Design review of the part built by this model. Coordinates are the model's own, in mm. A direction names the side the tool comes from. Coordinates: 2 decimals unless noted, no trailing zeros. Loops run counter-clockwise (first coordinate to the right, second up) from the corner with the lowest first, then second, coordinate; pieces in that order, holes last. Notation, with made-up numbers: (71, -16.5) - (104, -16.5) arc R16 ccw to (104, -11.5) - close; hole circle Ø3 at (66.5, 40). An arc over 180 degrees is marked (long way). Answer in a Markdown table with one row per item. Add a question column.
(1) For faces 5 (the face through (-9.75, 4, 0)), 6 (the face through (0, 9, 8)), 7 (the face through (-7.5, 11, 2.8)), list the 3-axis set-ups (+Z, -Z, +X, -X, +Y, -Y) from which the entire face can be reached by the end or side of a thin tool; tool diameter is ignored.
(2) We need section B-B, the plane y = 15.25. Write out the cut boundary in (x, z).
(3) We need section A-A, the plane y = 10.5. Write out the cut boundary in (x, z), plus the area to 3 significant figures.
(4) The part is to be moulded in two halves that separate along Y. For faces 1 (the face through (0, 5, 9.75)), 2 (the face through (0, 10.8, 8.2)), 3 (the face through (0, 10, 6.55)), 4 (the face through (0, 0, 0)), say which applies: released by +Y, released by -Y, zero draft, split by the parting line, or undercut.
(5) Clearance check with flat-ended pins moving along their axes: pin 1 (1.4 mm diameter, centred on x = 0, y = 10, fed in from +Z); pin 2 (1 mm diameter, centred on x = -7, y = 20, fed in from -Z); pin 3 (4 mm diameter, centred on y = 15.5, z = -1.5, fed in from -X). State where each tip first meets the part, or that it passes through.
(6) To check wall thickness, follow L1, parallel to Y at x = 0, z = 8.7; L2, parallel to Y at x = 0, z = 7.4; L3, parallel to Y at x = -5.5, z = 7.5. State the ranges of each line that lie inside material, in increasing order. Write a range as [from, to].
from build123d import *

# Parameters (mm, degrees)
SKETCH1_W           = 19.5
SKETCH1_H           = 19.5
BOSS_EXTRUDE1_DEPTH = 11
SKETCH2_R           = 7.75
BOSS_EXTRUDE2_DEPTH = 9
SKETCH3_R           = 7
BOSS_EXTRUDE3_DEPTH = 3.2
FILLET1_SIZE        = 1.5
FILLET1_SIZE_2      = 5
CHAMFER1_SIZE       = 2
BOSS_EXTRUDE8_REACH = 33.836
SKETCH4_R           = 3
SKETCH4_R_2         = 1
CUT_EXTRUDE1_DEPTH  = 3.2


# Some blends are built 0.0001 mm under size
with BuildPart() as part:
    # Sketch1 → Boss-Extrude1 (new body)
    with BuildSketch(Plane(origin=(0, 0, 0), x_dir=(1, 0, 0), z_dir=(0, 1, 0))):
        Rectangle(SKETCH1_W, SKETCH1_H)
    extrude(amount=BOSS_EXTRUDE1_DEPTH)

    # Sketch2 → Boss-Extrude2 (add)
    with BuildSketch(Plane(origin=(0, 11, 0), x_dir=(1, 0, 0), z_dir=(0, 1, 0))):
        with Locations(Location((0, 0, 0), (0, 0, 270))):
            Circle(SKETCH2_R)
    extrude(amount=BOSS_EXTRUDE2_DEPTH)

    # Sketch3 → Boss-Extrude3 (add)
    with BuildSketch(Plane(origin=(0, 20, 0), x_dir=(1, 0, 0), z_dir=(0, 1, 0))):
        with Locations(Location((0, 0, 0), (0, 0, 270))):
            Circle(SKETCH3_R)
    extrude(amount=BOSS_EXTRUDE3_DEPTH)

    # Fillet1
    # an asymmetric fillet: 5, 1.5 mm, written as the material it takes off along each edge
    with BuildSketch(Plane(origin=(0, 23.2, 0), x_dir=(0, 0, 1), z_dir=(-1, 0, 0))) as fillet1_piece_1:
        with BuildLine():
            Bezier((7, -FILLET1_SIZE), (7, 0), (7 - FILLET1_SIZE_2, 0), weights=[1, 0.707106781, 1])
            Line((7 - FILLET1_SIZE_2, 0), (7, 0))
            Line((7, 0), (7, -FILLET1_SIZE))
        make_face()
    revolve(axis=Axis((0, 23.2, 0), (0, 1, 0)), mode=Mode.SUBTRACT)

    # Chamfer1
    chamfer1_edges = [part.edges().sort_by_distance(p)[0] for p in [
        (-9.75, 11, 0),
        (0, 11, 9.75),
        (9.75, 11, 0),
        (0, 11, -9.75),
    ]]
    chamfer(chamfer1_edges, length=CHAMFER1_SIZE - 0.0001)  # a hair under: the kernel refuses the full size

    # Sketch4 → Boss-Extrude8 (add, up to next)
    with BuildSketch(Plane.XY.offset(9.75), mode=Mode.PRIVATE) as boss_extrude8_sk1:
        with Locations((0, 9.8)):
            Circle(SKETCH4_R)
        with Locations((0, 9.8)):
            Circle(SKETCH4_R_2, mode=Mode.SUBTRACT)
    boss_extrude8_tool1 = extrude(boss_extrude8_sk1.sketch, amount=-BOSS_EXTRUDE8_REACH, mode=Mode.PRIVATE) - part.part
    add(boss_extrude8_tool1.solids().sort_by_distance((-2.915147, 9.8, 9.75))[0])

    # Sketch5 → Cut-Extrude1 (cut)
    with BuildSketch(Plane.XY.offset(9.75)):
        with BuildLine():
            Line((0.6, 9), (-0.6, 9))
            ThreePointArc((-0.6, 9), (0, 10.8), (0.6, 9))
        make_face()
    extrude(amount=-CUT_EXTRUDE1_DEPTH, mode=Mode.SUBTRACT)


solid = part.part
Responses:
| question | item | result |
|---|---|---|
| 1 | face 5 | +Z, -Z, -X, +Y, -Y |
| 1 | face 6 | +Z |
| 1 | face 7 | +Y |
| 2 | outline | circle Ø15.5 at (0, 0) |
| 3 | outline | (-8.25, -8.25) - (8.25, -8.25) - (8.25, 8.25) - (2.92, 8.25) - (2.92, 9.75) - (0.71, 9.75) - (0.71, 6.55) - (-0.71, 6.55) - (-0.71, 9.75) - (-2.92, 9.75) - (-2.92, 8.25) - (-8.25, 8.25) - close |
| 3 | area | 276 mm2 |
| 4 | face 1 | zero draft |
| 4 | face 2 | undercut |
| 4 | face 3 | undercut |
| 4 | face 4 | released by -Y |
| 5 | pin 1 | stops at z = 6.55 |
| 5 | pin 2 | stops at z = -4.22 |
| 5 | pin 3 | stops at x = -7.75 |
| 6 | L1 | y = [0, 9], [10.8, 12.8] |
| 6 | L2 | y = [0, 9], [10.8, 20] |
| 6 | L3 | y = [0, 11] |
